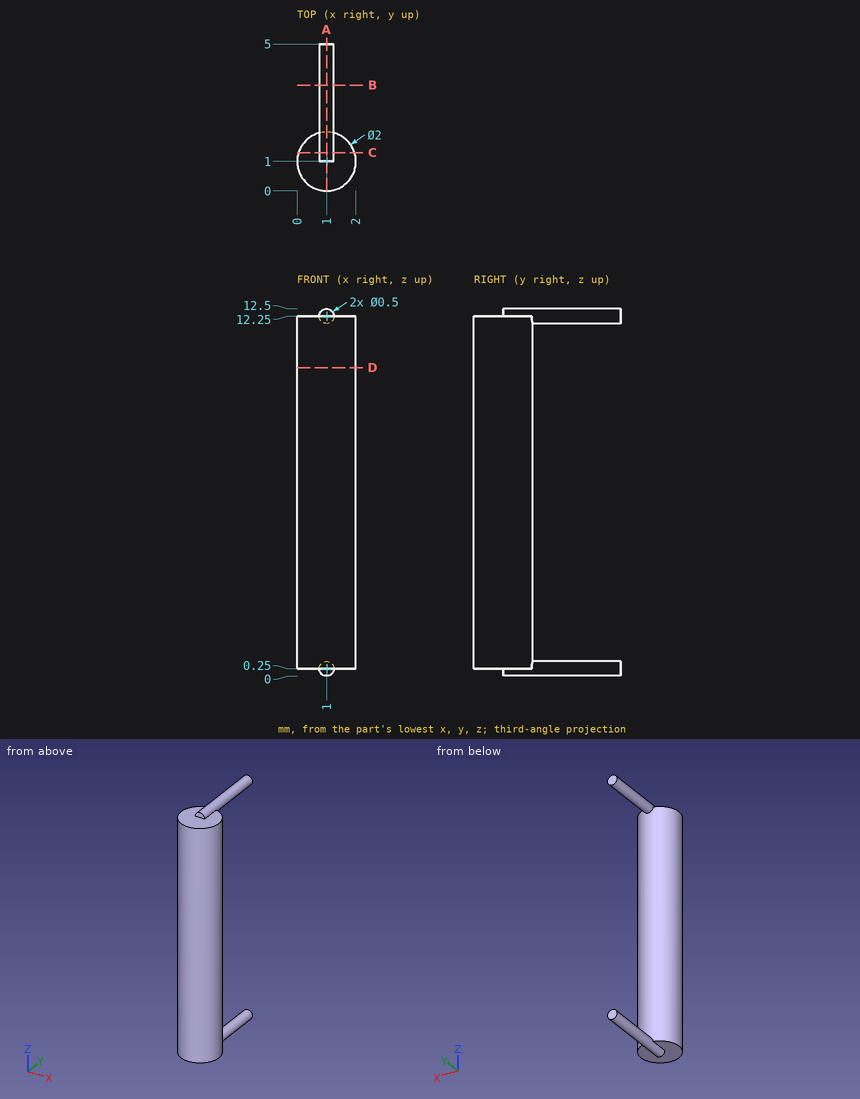
Verification items for this drawing (mm, ordinates from the low corner). Coordinates: 2 decimals unless noted, no trailing zeros. Loops run counter-clockwise (first coordinate to the right, second up) from the corner with the lowest first, then second, coordinate; pieces in that order, holes last.
Item 1: Sectioned sample at C-C, the plane y = 1.3. Record the boundary of the cut face in (x, z).
Item 2: Sectioned sample at D-D, the plane z = 10.5. Record the boundary of the cut face in (x, y), then the cut area to 3 significant figures.
Item 3: Thickness scan on line 1 (Z direction, x = 1.3, y = 1.1); line 2 (Z direction, x = 1.15, y = 3.9); line 3 (X direction, y = 1.35, z = 7.25). Record the ranges inside material, lowest first.
Item 4: Sectioned sample at B-B, the plane y = 3.6. Record the boundary of the cut face in (x, z).
Item 5: Sectioned sample at A-A, the plane x = 1. Record the boundary of the cut face in (y, z).
Check result:
1. outline: (0.05, 0.25) - (0.75, 0.25) arc R0.25 ccw to (1.25, 0.25) - (1.95, 0.25) - (1.95, 12.25) - (1.25, 12.25) arc R0.25 ccw to (0.75, 12.25) - (0.05, 12.25) - close
2. outline: circle Ø2 at (1, 1)
2. area: 3.14 mm2
3. line 1: z = 0.25 to 12.25
3. line 2: z = 0.05 to 0.45, 12.05 to 12.45
3. line 3: x = 0.06 to 1.94
4. outline: circle Ø0.5 at (1, 0.25); circle Ø0.5 at (1, 12.25)
5. outline: (0, 0.25) - (1, 0.25) - (1, 0) - (5, 0) - (5, 0.5) - (2, 0.5) - (2, 12) - (5, 12) - (5, 12.5) - (1, 12.5) - (1, 12.25) - (0, 12.25) - close
